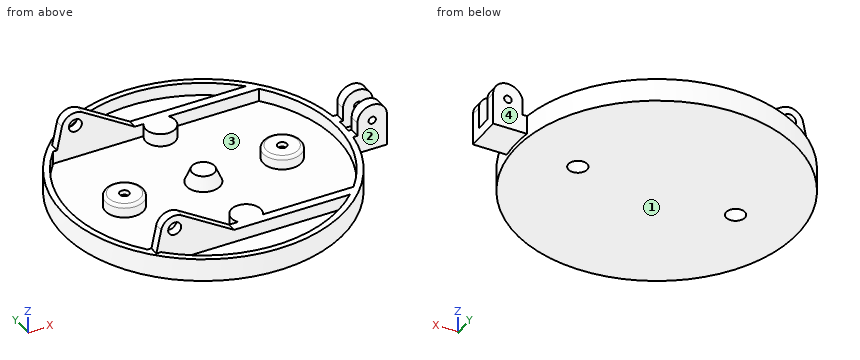
```python
from build123d import *

# Parameters (mm, degrees)
ESQUISSE1_R                  = 92.5
BOSS_EXTRU_1_DEPTH           = 15.1
ESQUISSE2_R                  = 88.5
ENL_V_MAT_EXTRU_1_DEPTH      = 8.5
BOSS_EXTRU_2_DEPTH           = 8.5
ESQUISSE4_R                  = 11
BOSS_EXTRU_3_DEPTH           = 8.5
BOSS_EXTRU_3_TAPER           = 23
BOSS_EXTRU_4_DEPTH           = 12.2
ENL_V_MAT_EXTRU_2_REACH      = 230.654
ENL_V_MAT_EXTRU_2_END_RADIUS = 92.5
ESQUISSE6_W                  = 23.8
ESQUISSE6_H                  = 10.4
TROU_TARAUD_M61_D            = 5
TROU_TARAUD_M61_DEPTH        = 13
TROU_TARAUD_M61_TIP          = 1.502151548
ESQUISSE9_R                  = 2.375
ENL_V_MAT_EXTRU_3_DEPTH      = 154.76638937
ESQUISSE10_R                 = 4.25
BOSS_EXTRU_5_DEPTH           = 6
ESQUISSE11_R                 = 12.5
BOSS_EXTRU_6_DEPTH           = 8.5
CONG_1_R                     = 2
R_P_TITION_CIRCULAIRE1_COUNT = 2


with BuildPart() as part:
    # Esquisse1 → Boss.-Extru.1 (new body)
    with BuildSketch(Plane.XY):
        Circle(ESQUISSE1_R)
    extrude(amount=BOSS_EXTRU_1_DEPTH)

    # Esquisse2 → Enlèv. mat.-Extru.1 (cut)
    with BuildSketch(Plane.XY.offset(15.1)):
        Circle(ESQUISSE2_R)
    extrude(amount=-ENL_V_MAT_EXTRU_1_DEPTH, mode=Mode.SUBTRACT)

    # Esquisse3 → Boss.-Extru.2 (add)
    with BuildSketch(Plane.XY.offset(15.1)):
        with BuildLine():
            Line((-62.01282448, 63.14), (62.01282448, 63.14))
            ThreePointArc((62.01282448, 63.14), (64.86661415, 60.204421504), (67.58158329, 57.14))
            Line((67.58158329, 57.14), (8.215838363, 57.14))
            ThreePointArc((8.215838363, 57.14), (0, 42.14), (-8.215838363, 57.14))
            Line((-8.215838363, 57.14), (-67.58158329, 57.14))
            ThreePointArc((-67.58158329, 57.14), (-64.86661415, 60.204421504), (-62.01282448, 63.14))
        make_face()
        with BuildLine():
            Line((-67.58158329, -57.14), (-8.215838363, -57.14))
            ThreePointArc((-8.215838363, -57.14), (0, -42.14), (8.215838363, -57.14))
            Line((8.215838363, -57.14), (67.58158329, -57.14))
            ThreePointArc((67.58158329, -57.14), (64.86661415, -60.204421504), (62.01282448, -63.14))
            Line((62.01282448, -63.14), (-62.01282448, -63.14))
            ThreePointArc((-62.01282448, -63.14), (-64.86661415, -60.204421504), (-67.58158329, -57.14))
        make_face()
    extrude(amount=-BOSS_EXTRU_2_DEPTH)

    # Esquisse4 → Boss.-Extru.3 (add)
    with BuildSketch(Plane.XY.offset(6.6)):
        Circle(ESQUISSE4_R)
    extrude(amount=BOSS_EXTRU_3_DEPTH, taper=BOSS_EXTRU_3_TAPER)

    # Esquisse5 → Boss.-Extru.4 (add, symmetric)
    with BuildSketch(Plane(origin=(0, 0, 0), x_dir=(1, 0, 0), z_dir=(0, 1, 0))):
        with BuildLine():
            Line((90.5, -2.75), (113.9, -2.75))
            Line((113.9, -2.75), (113.9, -23.85))
            ThreePointArc((113.9, -23.85), (104.2, -33.55), (94.5, -23.85))
            Line((94.5, -23.85), (94.5, -15.1))
            Line((94.5, -15.1), (90.5, -15.1))
            Line((90.5, -15.1), (90.5, -2.75))
        make_face()
    extrude(amount=BOSS_EXTRU_4_DEPTH, both=True)

    # Enlèv. mat.-Extru.2: up to this cylinder (the profile starts outside it)
    enl_v_mat_extru_2_end = Plane(origin=(0, 0, 21.65), z_dir=(0, 0, -1)) * Cylinder(ENL_V_MAT_EXTRU_2_END_RADIUS, 647.308, mode=Mode.PRIVATE)
    # Esquisse6 → Enlèv. mat.-Extru.2 (cut, up to the surface)
    with BuildSketch(Plane(origin=(113.9, 0, 0), x_dir=(0, 0, -1), z_dir=(1, 0, 0)), mode=Mode.PRIVATE) as enl_v_mat_extru_2_sk1:
        with Locations((-21.65, 0)):
            Rectangle(ESQUISSE6_W, ESQUISSE6_H)
    enl_v_mat_extru_2_tool1 = extrude(enl_v_mat_extru_2_sk1.sketch, amount=-ENL_V_MAT_EXTRU_2_REACH, mode=Mode.PRIVATE) - enl_v_mat_extru_2_end
    add(enl_v_mat_extru_2_tool1.solids().sort_by_distance((113.9, 0, 21.65))[0], mode=Mode.SUBTRACT)

    # Trou taraudé M61
    with Locations(Plane(origin=(0, 12.2, 0), x_dir=(-1, 0, 0), z_dir=(0, 1, 0))):
        with Locations((-104.2, 22.75)):
            Hole(TROU_TARAUD_M61_D / 2, depth=TROU_TARAUD_M61_DEPTH)
            with Locations((0, 0, -(TROU_TARAUD_M61_DEPTH + TROU_TARAUD_M61_TIP / 2))):  # 118° drill point
                Cone(0, TROU_TARAUD_M61_D / 2, TROU_TARAUD_M61_TIP, mode=Mode.SUBTRACT)

    # Esquisse9 → Enlèv. mat.-Extru.3 (cut, through all)
    with BuildSketch(Plane(origin=(0, -5.2, 0), x_dir=(1, 0, 0), z_dir=(0, 1, 0))):
        with Locations(Location((104.2, -22.75, 0), (0, 0, 270))):
            Circle(ESQUISSE9_R)
    extrude(amount=-ENL_V_MAT_EXTRU_3_DEPTH, mode=Mode.SUBTRACT)

    # Esquisse10 → Boss.-Extru.5 (add)
    with BuildSketch(Plane(origin=(0, 63.14, 0), x_dir=(1, 0, 0), z_dir=(0, 1, 0))):
        with BuildLine():
            Line((-14, -15.1), (-48.272170546, -36.258173977))
            ThreePointArc((-48.272170546, -36.258173977), (-56.557229613, -36.867171069), (-61.811481567, -30.43242806))
            Line((-61.811481567, -30.43242806), (-65, -15.1))
            Line((-65, -15.1), (-14, -15.1))
        make_face()
        with Locations(Location((-53, -28.6, 0), (0, 0, 270))):
            Circle(ESQUISSE10_R, mode=Mode.SUBTRACT)
    boss_extru_5 = extrude(amount=-BOSS_EXTRU_5_DEPTH)

    # Symétrie1: Boss.-Extru.5 across plane
    add(boss_extru_5.mirror(Plane.ZX))

    # Esquisse11 → Boss.-Extru.6 (add)
    with BuildSketch(Plane.XY.offset(6.6)):
        with Locations((-51.75, 0)):
            Circle(ESQUISSE11_R)
        with Locations((51.75, 0)):
            Circle(ESQUISSE11_R)
    extrude(amount=BOSS_EXTRU_6_DEPTH)

    # Congé1
    cong_1_edges = [part.edges().sort_by_distance(p)[0] for p in [
        (-64.25, 0, 15.1),
        (39.25, 0, 15.1),
    ]]
    fillet(cong_1_edges, radius=CONG_1_R)

    # Esquisse12 → Enlèvement de matière-Révolution1 (revolve, cut)
    with BuildSketch(Plane(origin=(0, 0, 0), x_dir=(1, 0, 0), z_dir=(0, 1, 0)), mode=Mode.PRIVATE) as enl_vement_de_mati_re_r_volution1_sk:
        Polygon((57.9, 0), (57.9, -12), (54.85, -12), (54.85, -15.1), (51.75, -15.1), (51.75, 0), align=None)
    enl_vement_de_mati_re_r_volution1 = revolve(enl_vement_de_mati_re_r_volution1_sk.sketch.rotate(Axis((51.75, 0, -5.611731472), (0, 0, 1)), 180), axis=Axis((51.75, 0, -5.611731472), (0, 0, 1)), mode=Mode.SUBTRACT)

    # Répétition circulaire1: Enlèvement de matière-Révolution1 ×2 about axis
    r_p_tition_circulaire1_axis = Axis((0, 0, 0), (0, 0, 1))
    for i in range(1, R_P_TITION_CIRCULAIRE1_COUNT):
        add(enl_vement_de_mati_re_r_volution1.rotate(r_p_tition_circulaire1_axis, i * 360 / R_P_TITION_CIRCULAIRE1_COUNT), mode=Mode.SUBTRACT)


solid = part.part
```
Can you work these out from the model? Positions are in its coordinate system, mm. Face numbers are marked on the shaded views. Coordinates: 2 decimals unless noted, no trailing zeros. Loops run counter-clockwise (first coordinate to the right, second up) from the corner with the lowest first, then second, coordinate; pieces in that order, holes last. Notation, with made-up numbers: (85, -21.75) - (129, -21.75) arc R23 ccw to (129, -0.75) - close; hole circle Ø3 at (-13, 10.25). An arc over 180 degrees is marked (long way). Answer as CSV lines item,"result". Start each with the question number.
1) Suppose I cut it at A-A (x = 0). Please give me the cut outline in (y, z).
2) I need wall thicknesses on line 1 (Y direction, x = -53, z = 19.5); line 2 (Y direction, x = 43, z = 14); line 3 (Y direction, x = -51.75, z = 13.45). Which ranges of each line are inside material? Lowest first, please. Write a range as from..to.
3) Suppose I cut it at D-D (x = -70.5). Please give me the cut outline in (y, z).
4) For pin 1 (15.5 mm diameter, centred on x = -30.5, z = 24.5, fed in from -Y); pin 2 (10 mm diameter, centred on x = -49, y = 0.5, fed in from -Z); pin 3 (18 mm diameter, centred on x = 106, z = 18, fed in from -Y); pin 4 (6.5 mm diameter, centred on x = -49.5, y = 0, fed in from +Z), each with a flat end and sliding along its axis, tell me the tip position at first contact or that it passes through.
5) Suppose I cut it at B-B (y = -20). Please give me the cut outline in (x, z).
6) Thinking about a two-plate mould opening in Y: for the marked faces 1, 2, 3 and 4, which applies, pulls with the +Y half, pulls with the -Y half, needs draft (parallel to the pull), parting line crosses it, or undercut?
7) Suppose I cut it at C-C (y = 0). Count the separate pieces of the cut face and the enclosed holes in it, plus the area to 3 significant figures.
Check result:
1,outline,"(-92.5, 0) - (92.5, 0) - (92.5, 15.1) - (88.5, 15.1) - (88.5, 6.6) - (63.14, 6.6) - (63.14, 15.1) - (42.14, 15.1) - (42.14, 6.6) - (11, 6.6) - (7.39, 15.1) - (-7.39, 15.1) - (-11, 6.6) - (-42.14, 6.6) - (-42.14, 15.1) - (-63.14, 15.1) - (-63.14, 6.6) - (-88.5, 6.6) - (-88.5, 15.1) - (-92.5, 15.1) - close"
2,line 1,"y = -63.14..-57.14, 57.14..63.14"
2,line 2,"y = -81.9..-77.35, -63.14..-57.14, -8.62..8.62, 57.14..63.14, 77.35..81.9"
2,line 3,"y = -76.67..-71.79, -63.14..-57.14, -12.47..-3.1, 3.1..12.47, 57.14..63.14, 71.79..76.67"
3,outline,"(-59.88, 0) - (59.88, 0) - (59.88, 15.1) - (53.5, 15.1) - (53.5, 6.6) - (-53.5, 6.6) - (-53.5, 15.1) - (-59.88, 15.1) - close"
4,pin 1,"stops at y = -63.14"
4,pin 2,"stops at z = 0"
4,pin 3,"stops at y = -12.2"
4,pin 4,"stops at z = 15.1"
5,outline,"(-90.31, 0) - (90.31, 0) - (90.31, 15.1) - (86.21, 15.1) - (86.21, 6.6) - (-86.21, 6.6) - (-86.21, 15.1) - (-90.31, 15.1) - close"
6,face 1,"needs draft"
6,face 2,"pulls with the -Y half"
6,face 3,"undercut"
6,face 4,"pulls with the +Y half"
7,separate pieces,"3"
7,enclosed holes,"0"
7,area,"1,680 mm²"
